Geometry: final body of the model. Coordinates: model frame, mm. Face numbers are marked on the shaded views. Give positions to 0.01 mm unless a question says otherwise; leave off trailing zeros. Loops run counter-clockwise (first coordinate to the right, second up) from the corner with the lowest first, then second, coordinate; pieces in that order, holes last. Notation, with made-up numbers: M 60,11 L 110,11 A15 cw 110,27 Z; hole C 0,42 d1. An arc over 180 degrees is marked long. One line per question, with ' | ' between items. Start each with the question number.
from build123d import *

# Parameters (mm, degrees)
F0_R      = 62
F1_DEPTH  = 17
F2_R      = 60
F3_DEPTH  = 15
F4_R      = 14.99999
F5_R      = 61
F6_DEPTH  = 4
F8_DEPTH  = 25
F9_R      = 3
F10_R     = 8
F11_DEPTH = 25


# Not quite as in the source:
# - a fillet or chamfer is up to 0.001 mm smaller than in the source, because OpenCascade refuses the exact size


with BuildPart() as f1:
    # F0 (on Top) → F1 (new body)
    with BuildSketch(Plane.XY):
        Circle(F0_R)
    extrude(amount=F1_DEPTH)

    # F2 (on face) → F3 (cut)
    with BuildSketch(Plane(origin=(0, 0, 0), x_dir=(1, 0, 0), z_dir=(0, 0, -1))):
        Circle(F2_R)
    extrude(amount=-F3_DEPTH, mode=Mode.SUBTRACT)

    # F4 (radius 15 in the source; OpenCascade refuses exactly that, so slightly less here)
    f4_edges = [f1.edges().sort_by_distance(p)[0] for p in [
        (-60, 0, 15),
        (-62, 0, 17),
    ]]
    fillet(f4_edges, radius=F4_R)

    # F5 (on face) → F6 (cut)
    with BuildSketch(Plane(origin=(0, 0, 0), x_dir=(1, 0, 0), z_dir=(0, 0, -1))):
        Circle(F5_R)
    extrude(amount=-F6_DEPTH, mode=Mode.SUBTRACT)

    # F7 (on face) → F8 (cut)
    with BuildSketch(Plane.XY.offset(17)):
        with BuildLine():
            Line((-43.1747773956, -18.5725479362), (-12, 0))
            Line((-12, 0), (-43.1747773956, 18.5725479362))
            ThreePointArc((-43.1747773956, 18.5725479362), (-47.00001, 0), (-43.1747773956, -18.5725479362))
        make_face()
        with BuildLine():
            ThreePointArc((-43.1747773956, -18.5725479362), (-47.00001, 0), (-43.1747773956, 18.5725479362))
            Line((-43.1747773956, 18.5725479362), (-53.2366762866, 24.5669804581))
            ThreePointArc((-53.2366762866, 24.5669804581), (-58.8026071187, 0), (-53.2366762866, -24.5669804581))
            Line((-53.2366762866, -24.5669804581), (-43.1747773956, -18.5725479362))
        make_face()
    extrude(amount=-F8_DEPTH, mode=Mode.SUBTRACT)

    # F9
    f9_edges = [f1.edges().sort_by_distance(p)[0] for p in [
        (-12, 0, 16),
        (-53.236676, -24.56698, 8.865114),
        (-53.236676, 24.56698, 8.865114),
    ]]
    fillet(f9_edges, radius=F9_R)

    # F10 (on face) → F11 (cut)
    with BuildSketch(Plane.XY.offset(17)):
        Circle(F10_R)
    extrude(amount=-F11_DEPTH, mode=Mode.SUBTRACT)


solid = f1.part
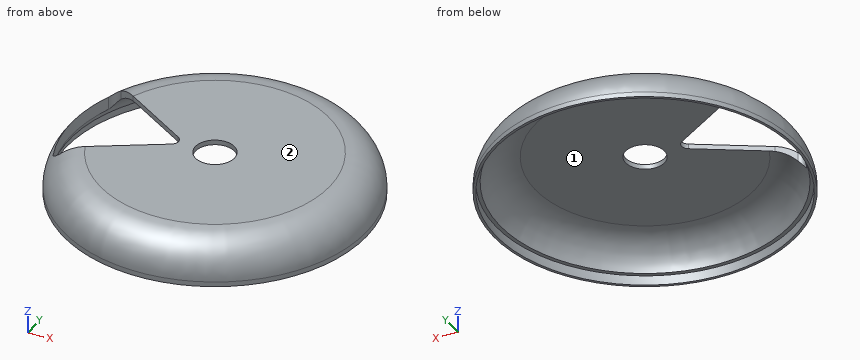
Q1. Contact query for flat-ended pins moving along their axis: pin 1 (3 mm diameter, centred on x = 28, y = 0.5, fed in from -Z); pin 2 (3 mm diameter, centred on x = -18, z = 2, fed in from +Y); pin 3 (14.5 mm diameter, centred on x = 0, y = 0, fed in from +Z); pin 4 (2 mm diameter, centred on y = 40, z = 6, fed in from -X). Output: stop coordinate, or through.
Q2. Section A-A, the plane x = 0. Output: boundary loops of the cut face in (y, z), plus the area to 3 significant figures.
Q3. Section C-C, the plane z = 8.5. Output: boundary loops of the cut face in (x, y), plus the area to 3 significant figures.
Q4. Section B-B, the plane y = 0. Output: boundary loops of the cut face in (x, z).
Q5. Material intervals for L1, parallel to Y at x = 0, z = 0.85; L2, parallel to Z at x = 4.5, y = -20.5; L3, parallel to Y at x = 54, z = 5.25, sorted ascending.
Q6. Draft query along Y for the marked faces 1 and 2. Return one class per face: released by +Y, released by -Y, zero draft, split by the parting line, or undercut.
Model answer:
1) pin 1: stops at z = 15 | pin 2: stops at y = 59.76 | pin 3: passes through | pin 4: stops at x = -47.56
2) outline: M -62,0 L -61,0 L -61,4 L -59.46,4 A15 cw -45,15 L -8,15 L -8,17 L -47,17 A15 ccw -62,2 Z; M 8,15 L 45,15 A15 cw 59.46,4 L 61,4 L 61,0 L 62,0 L 62,2 A15 ccw 47,17 L 8,17 Z | area: 267 mm^2
3) outline: C 0,0 d121.04; hole M -54.64,-21.38 A3 ccw -52.46,-23.19 A57.36 ccw long -52.46,23.19 A3 ccw -54.64,21.38 A57 ccw Z | area: 1,100 mm^2
4) outline: M -62,0 L -61,0 L -61,4 L -59.46,4 A15 cw -58.8,5.87 L -58.8,11.26 A15 ccw -62,2 Z; M -14.86,15 L -8,15 L -8,17 L -14.86,17 Z; M 8,15 L 45,15 A15 cw 59.46,4 L 61,4 L 61,0 L 62,0 L 62,2 A15 ccw 47,17 L 8,17 Z
5) L1: y = -62 to -61, 61 to 62 | L2: z = 15 to 17 | L3: y = -29.73 to -23.9, 23.9 to 29.73
6) face 1: undercut | face 2: zero draft
